The drawing under review shows one solid part. Ordinate dimensions are in mm from its lowest x, y, z. Round coordinates to 2 decimals unless told otherwise and drop trailing zeros. Write each loop counter-clockwise with the first axis right and the second up, starting at its lowest first coordinate (ties: lowest second). Pieces come first, ordered by that corner, then holes.
Item 1: Add section B-B (x = 5). Give the boundary of the cut face in (y, z).
Item 2: Add section C-C (y = 1.75). Give the boundary of the cut face in (x, z).
Item 3: To check wall thickness, follow L1, parallel to Z at x = 5, y = 3.5; L2, parallel to Z at x = 6, y = 6.25; L3, parallel to X at y = 0.5, z = 11.5. State the ranges of each line that lie inside material, in increasing order.
Item 4: Draft analysis for pull direction Z (two halves, no side actions). For the marked faces 1, 2 and 3, state which applies: +Z half, -Z half, draft (parallel to the pull), parting line (faces both ways), or undercut.
Item 5: Add section A-A (z = 10). Give the boundary of the cut face in (x, y).
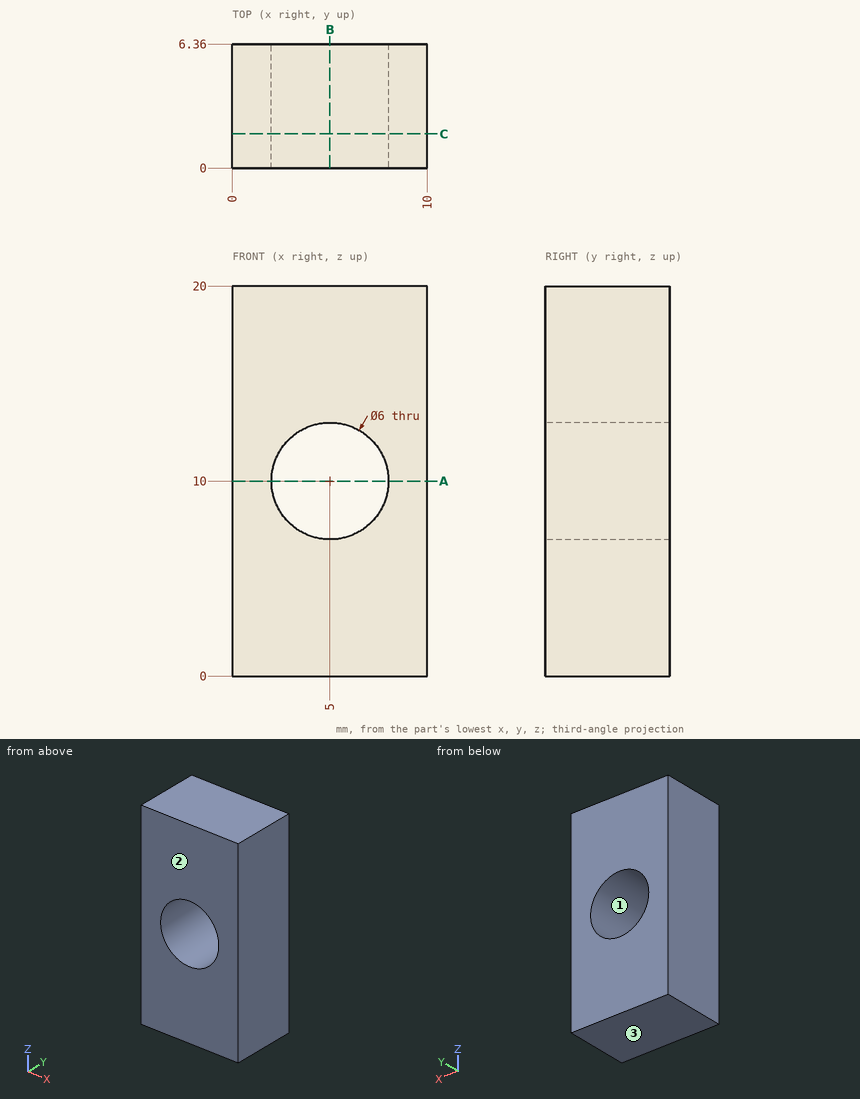
Numbers:
1. outline: (0, 0) - (6.36, 0) - (6.36, 7) - (0, 7) - close; (0, 13) - (6.36, 13) - (6.36, 20) - (0, 20) - close
2. outline: (0, 0) - (10, 0) - (10, 20) - (0, 20) - close; hole circle Ø6 at (5, 10)
3. L1: z = 0 to 7, 13 to 20
3. L2: z = 0 to 7.17, 12.83 to 20
3. L3: x = 0 to 2.4, 7.6 to 10
4. face 1: undercut
4. face 2: draft
4. face 3: -Z half
5. outline: (0, 0) - (2, 0) - (2, 6.36) - (0, 6.36) - close; (8, 0) - (10, 0) - (10, 6.36) - (8, 6.36) - close
